```python
from build123d import *

# Parameters (mm, degrees)
F2_W      = 9
F2_H      = 83
F3_DEPTH  = 63
F4_R      = 2.85
F5_DEPTH  = 3.5
F6_R      = 1.6
F7_DEPTH  = 25
F8_W      = 17
F8_H      = 45
F9_DEPTH  = 20
F11_DEPTH = 70
F12_W     = 8
F12_H     = 45
F13_DEPTH = 9
F14_DEPTH = 5
F15_R     = 2.85
F16_DEPTH = 3.5
F17_R     = 1.6
F18_DEPTH = 25
F20_DEPTH = 3
F21_W     = 9
F21_H     = 40.2
F22_DEPTH = 24
F23_W     = 24
F23_H     = 4.8
F24_DEPTH = 2
F25_SIZE  = 1.5
F26_R     = 1.6
F27_DEPTH = 25
F28_R     = 1.6
F29_DEPTH = 25
F30_W     = 29
F30_H     = 4.8
F31_DEPTH = 2
F32_SIZE  = 1.5
F33_DEPTH = 3
F34_W     = 24
F34_H     = 4.8
F35_DEPTH = 2
F36_SIZE  = 1.5
F37_R     = 1.6
F38_DEPTH = 25
F39_W     = 24
F39_H     = 4.8
F40_DEPTH = 2
F41_SIZE  = 1.5
F42_R     = 1.6
F43_DEPTH = 25
F44_R     = 2.85
F45_DEPTH = 3.5
F46_R     = 2.85
F47_DEPTH = 3.5
F48_R     = 5
F49_R     = 5
F50_R     = 5
F51_R     = 2.85
F51_R_2   = 1.6
F52_DEPTH = 3.5


with BuildPart() as f3:
    # F2 (on Top) → F3 (new body)
    with BuildSketch(Plane.XY):
        with Locations((4.5, 41.5)):
            Rectangle(F2_W, F2_H)
    extrude(amount=F3_DEPTH)

    # F4 (on face) → F5 (cut)
    with BuildSketch(Plane.YZ.offset(9)):
        with Locations((8.5, 40.5)):
            Circle(F4_R)
        with Locations((8.5, 22.5)):
            Circle(F4_R)
        with Locations((78, 56.5)):
            Circle(F4_R)
        with Locations((78, 38.5)):
            Circle(F4_R)
        with Locations((78, 24.5)):
            Circle(F4_R)
        with Locations((78, 6.5)):
            Circle(F4_R)
    extrude(amount=-F5_DEPTH, mode=Mode.SUBTRACT)

    # F6 (on face) → F7 (cut)
    with BuildSketch(Plane.YZ.offset(9)):
        with Locations((8.5, 40.5)):
            Circle(F6_R)
        with Locations((8.5, 22.5)):
            Circle(F6_R)
        with Locations((78, 24.5)):
            Circle(F6_R)
        with Locations((78, 38.5)):
            Circle(F6_R)
        with Locations((78, 56.5)):
            Circle(F6_R)
        with Locations((78, 6.5)):
            Circle(F6_R)
    extrude(amount=-F7_DEPTH, mode=Mode.SUBTRACT)

    # F8 (on face) → F9 (join)
    with BuildSketch(Plane.YZ.offset(9)):
        with Locations((64.5, 31.5)):
            Rectangle(F8_W, F8_H)
    extrude(amount=F9_DEPTH)

    # F10 (on face) → F11 (cut)
    with BuildSketch(Plane.XY.offset(54)):
        Polygon((28.6786117956, 64.5474786816), (24.7981881534, 71.1736122216), (17.1195763578, 71.12613354), (13.3213882044, 64.4525213184), (17.2018118466, 57.8263877784), (24.8804236422, 57.87386646), align=None)
    extrude(amount=-F11_DEPTH, mode=Mode.SUBTRACT)

    # F12 (on face) → F13 (join)
    with BuildSketch(Plane.YZ.offset(29)):
        with Locations((69, 31.5)):
            Rectangle(F12_W, F12_H)
        with Locations((60, 31.5)):
            Rectangle(F12_W, F12_H)
    extrude(amount=F13_DEPTH)

    # F14 (cut): a face of the model
    f14_faces = [f3.faces().sort_by_distance(p)[0] for p in [
        (29, 64.5, 31.5),
    ]]
    extrude(f14_faces, amount=-F14_DEPTH, mode=Mode.SUBTRACT)

    # F15 (on face) → F16 (cut)
    with BuildSketch(Plane.XZ.offset(-56)):
        with Locations((34.5, 46)):
            Circle(F15_R)
        with Locations((34.5, 31.5)):
            Circle(F15_R)
        with Locations((34.5, 17)):
            Circle(F15_R)
    extrude(amount=-F16_DEPTH, mode=Mode.SUBTRACT)

    # F17 (on face) → F18 (cut)
    with BuildSketch(Plane.XZ.offset(-59.5)):
        with Locations((34.5, 46)):
            Circle(F17_R)
        with Locations((34.5, 31.5)):
            Circle(F17_R)
        with Locations((34.5, 17)):
            Circle(F17_R)
    extrude(amount=-F18_DEPTH, mode=Mode.SUBTRACT)

    # F19 (on face) → F20 (cut)
    with BuildSketch(Plane(origin=(0, 73, 0), x_dir=(-1, 0, 0), z_dir=(0, 1, 0))):
        Polygon((-32.8545517328, 48.85), (-36.1454482672, 48.85), (-37.7908965344, 46), (-36.1454482672, 43.15), (-32.8545517328, 43.15), (-31.2091034656, 46), align=None)
        Polygon((-37.7908965344, 31.5), (-36.1454482672, 28.65), (-32.8545517328, 28.65), (-31.2091034656, 31.5), (-32.8545517328, 34.35), (-36.1454482672, 34.35), align=None)
        Polygon((-31.2091034656, 17), (-32.8545517328, 19.85), (-36.1454482672, 19.85), (-37.7908965344, 17), (-36.1454482672, 14.15), (-32.8545517328, 14.15), align=None)
    extrude(amount=-F20_DEPTH, mode=Mode.SUBTRACT)

    # F21 (on face) → F22 (join)
    with BuildSketch(Plane.YZ.offset(9)):
        with Locations((31.3, 31.5)):
            Rectangle(F21_W, F21_H)
        Polygon((26.8, 51.6), (35.8, 51.6), (56, 51.6), (56, 60.6), (26.8, 60.6), align=None)
        Polygon((56, 11.4), (35.8, 11.4), (26.8, 11.4), (26.8, 2.4), (56, 2.4), align=None)
    extrude(amount=F22_DEPTH)

    # F23 (on face) → F24 (join)
    with BuildSketch(Plane(origin=(0, 35.8, 0), x_dir=(-1, 0, 0), z_dir=(0, 1, 0))):
        with Locations((-21, 41.5)):
            Rectangle(F23_W, F23_H)
        with Locations((-21, 21.5)):
            Rectangle(F23_W, F23_H)
    extrude(amount=F24_DEPTH)

    # F25
    f25_edges = [f3.edges().sort_by_distance(p)[0] for p in [
        (21, 37.8, 39.1),
        (21, 37.8, 43.9),
        (21, 37.8, 23.9),
        (21, 37.8, 19.1),
    ]]
    chamfer(f25_edges, length=F25_SIZE)

    # F26 (on face) → F27 (cut)
    with BuildSketch(Plane(origin=(0, 37.8, 0), x_dir=(-1, 0, 0), z_dir=(0, 1, 0))):
        with Locations((-21, 41.5)):
            Circle(F26_R)
        with BuildLine():
            Line((-22.3228756555, 42.4), (-19.6771243445, 42.4))
            ThreePointArc((-19.6771243445, 42.4), (-21, 43.1), (-22.3228756555, 42.4))
        make_face()
    extrude(amount=-F27_DEPTH, mode=Mode.SUBTRACT)

    # F28 (on face) → F29 (cut)
    with BuildSketch(Plane(origin=(0, 37.8, 0), x_dir=(-1, 0, 0), z_dir=(0, 1, 0))):
        with Locations((-21, 21.5)):
            Circle(F28_R)
    extrude(amount=-F29_DEPTH, mode=Mode.SUBTRACT)

    # F30 (on face) → F31 (join)
    with BuildSketch(Plane.XZ.offset(-56)):
        with Locations((23.5, 21.5)):
            Rectangle(F30_W, F30_H)
        with Locations((23.5, 41.5)):
            Rectangle(F30_W, F30_H)
    extrude(amount=F31_DEPTH)

    # F32
    f32_edges = [f3.edges().sort_by_distance(p)[0] for p in [
        (23.5, 54, 43.9),
        (23.5, 54, 39.1),
        (23.5, 54, 23.9),
        (23.5, 54, 19.1),
    ]]
    chamfer(f32_edges, length=F32_SIZE)

    # F15 (on face) → F33 (cut)
    with BuildSketch(Plane.XZ.offset(-56)):
        with Locations((34.5, 46)):
            Circle(F15_R)
        with Locations((34.5, 31.5)):
            Circle(F15_R)
        with Locations((34.5, 17)):
            Circle(F15_R)
    extrude(amount=F33_DEPTH, mode=Mode.SUBTRACT)

    # F34 (on face) → F35 (join)
    with BuildSketch(Plane(origin=(0, 0, 51.6), x_dir=(1, 0, 0), z_dir=(0, 0, -1))):
        with Locations((21, -45.9)):
            Rectangle(F34_W, F34_H)
    extrude(amount=F35_DEPTH)

    # F36
    f36_edges = [f3.edges().sort_by_distance(p)[0] for p in [
        (21, 43.5, 49.6),
        (21, 48.3, 49.6),
    ]]
    chamfer(f36_edges, length=F36_SIZE)

    # F37 (on face) → F38 (cut)
    with BuildSketch(Plane(origin=(0, 0, 49.6), x_dir=(1, 0, 0), z_dir=(0, 0, -1))):
        with Locations((21, -45.9)):
            Circle(F37_R)
    extrude(amount=-F38_DEPTH, mode=Mode.SUBTRACT)

    # F39 (on face) → F40 (join)
    with BuildSketch(Plane.XY.offset(11.4)):
        with Locations((21, 45.9)):
            Rectangle(F39_W, F39_H)
    extrude(amount=F40_DEPTH)

    # F41
    f41_edges = [f3.edges().sort_by_distance(p)[0] for p in [
        (21, 48.3, 13.4),
        (21, 43.5, 13.4),
    ]]
    chamfer(f41_edges, length=F41_SIZE)

    # F42 (on face) → F43 (cut)
    with BuildSketch(Plane.XY.offset(13.4)):
        with Locations((21, 45.9)):
            Circle(F42_R)
    extrude(amount=-F43_DEPTH, mode=Mode.SUBTRACT)

    # F44 (on face) → F45 (cut)
    with BuildSketch(Plane(origin=(0, 0, 2.4), x_dir=(1, 0, 0), z_dir=(0, 0, -1))):
        with Locations((21, -45.9)):
            Circle(F44_R)
    extrude(amount=-F45_DEPTH, mode=Mode.SUBTRACT)

    # F46 (on face) → F47 (cut)
    with BuildSketch(Plane.XZ.offset(-26.8)):
        with Locations((21, 41.5)):
            Circle(F46_R)
        with Locations((21, 21.5)):
            Circle(F46_R)
    extrude(amount=-F47_DEPTH, mode=Mode.SUBTRACT)

    # F48
    f48_edges = [f3.edges().sort_by_distance(p)[0] for p in [
        (21, 26.8, 2.4),
    ]]
    fillet(f48_edges, radius=F48_R)

    # F49
    f49_edges = [f3.edges().sort_by_distance(p)[0] for p in [
        (21, 26.8, 60.6),
    ]]
    fillet(f49_edges, radius=F49_R)

    # F50
    f50_edges = [f3.edges().sort_by_distance(p)[0] for p in [
        (21, 56, 2.4),
        (21, 56, 60.6),
    ]]
    fillet(f50_edges, radius=F50_R)

    # F51 (on face) → F52 (cut)
    with BuildSketch(Plane.XY.offset(60.6)):
        with Locations((21, 45.9)):
            Circle(F51_R)
        with Locations((21, 45.9)):
            Circle(F51_R_2, mode=Mode.SUBTRACT)
    extrude(amount=-F52_DEPTH, mode=Mode.SUBTRACT)


solid = f3.part
```
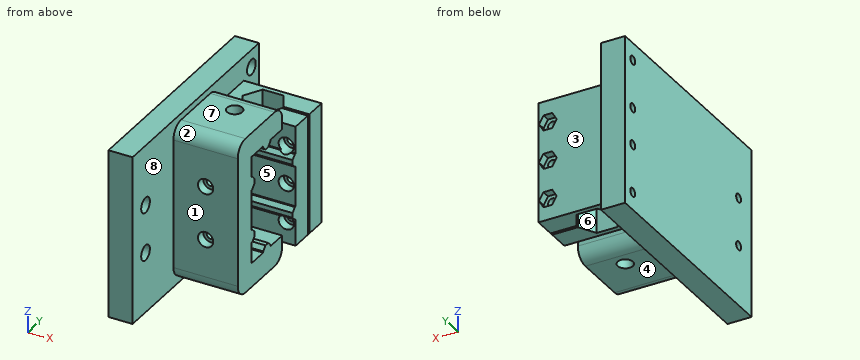
Geometry: final body of the model. Coordinates: model frame, mm. Face numbers are marked on the shaded views. A direction names the side the tool comes from. Round coordinates to 2 decimals unless told otherwise and drop trailing zeros. Loops run counter-clockwise (first coordinate to the right, second up) from the corner with the lowest first, then second, coordinate; pieces in that order, holes last. Notation, with made-up numbers: (27.5, -17) -> (68.5, -17) arc R22 ccw to (68.5, 21) -> close; hole circle Ø11 at (79.25, -19.75). An arc over 180 degrees is marked (long way). Use one line per item in the form item = value. Start each with the question number.
1) Section A-A on x = 8. Output: boundary loops of the cut face in (y, z), then the cut area to 3 significant figures.
2) Section B-B on y = 63. Output: boundary loops of the cut face in (x, z).
3) First-contact query: P1, Ø1.5, axis at x = 32.5, y = 28, coming from the -Z side; P2, Ø5, axis at x = 21, z = 41.5, coming from the -Y side; P3, Ø3.5, axis at y = 78, z = 6.5, coming from the -X side; P4, Ø2, axis at x = 28, y = 45.5, coming from the -Z side. Flat tips, straight axial feed; report the tip coordinate or a pass-through.
4) Section D-D on x = 26. Give the number of separate pieces and of enclosed holes in the cut face, then the cut area to 3 significant figures.
5) Access query for the marked faces 1, 2, 3, 4 and 5. Directions: +Z, -Z, +X, -X, +Y, -Y. A direction counts if a zero-diameter tool reaches every point of the face in a straight line with its end or side. Return the directions, or none.
6) Line query: L1, parallel to Z at x = 34.5, y = 68.25; L2, parallel to Z at x = 6.55, y = 78; L3, parallel to Y at x = 17.5, z = 25.5. Output: solid intervals per line, ascending.
7) Section C-C on y = 34. Output: boundary loops of the cut face in (x, z), then the cut area to 3 significant figures.
8) Draft query along X for the marked faces 6, 7 and 8. Return one class per face: released by +X, released by -X, zero draft, split by the parting line, or undercut.
Response:
q1.outline = (0, 0) -> (83, 0) -> (83, 63) -> (0, 63) -> close; hole circle Ø5.7 at (8.5, 22.5); hole circle Ø5.7 at (8.5, 40.5); hole circle Ø5.7 at (78, 6.5); hole circle Ø5.7 at (78, 24.5); hole circle Ø5.7 at (78, 38.5); hole circle Ø5.7 at (78, 56.5)
q1.area = 5,080 mm^2
q2.outline = (0, 0) -> (9, 0) -> (9, 9) -> (14.17, 9) -> (14.17, 54) -> (9, 54) -> (9, 63) -> (0, 63) -> close; (27.8, 9) -> (38, 9) -> (38, 54) -> (27.8, 54) -> close; hole circle Ø3.2 at (34.5, 17); hole circle Ø3.2 at (34.5, 31.5); hole circle Ø3.2 at (34.5, 46)
q3.P1 = 3.44
q3.P2 = 30.3
q3.P3 = 0
q3.P4 = 2.4
q4.separate_pieces = 2
q4.enclosed_holes = 1
q4.area = 1,260 mm^2
q5.face_1 = +Z, -Z, +X, -Y
q5.face_2 = +Z, +X, -Y
q5.face_3 = +Z, -Z, +X, +Y
q5.face_4 = -Z, +X, +Y, -Y
q5.face_5 = +X
q6.L1 = 9 to 15.4, 18.6 to 29.9, 33.1 to 44.4, 47.6 to 54
q6.L2 = 0 to 3.65, 9.35 to 21.65, 27.35 to 35.65, 41.35 to 53.65, 59.35 to 63
q6.L3 = 26.8 to 35.8, 56 to 57.83, 71.13 to 73
q7.outline = (0, 0) -> (9, 0) -> (9, 2.4) -> (33, 2.4) -> (33, 60.6) -> (9, 60.6) -> (9, 63) -> (0, 63) -> close; hole circle Ø3.2 at (21, 21.5); hole circle Ø3.2 at (21, 41.5)
q7.area = 1,950 mm^2
q8.face_6 = undercut
q8.face_7 = zero draft
q8.face_8 = released by +X
